Check sheet for the modelled part. Datum: model origin and axes. Units: mm. Give positions to 0.01 mm unless a question says otherwise; leave off trailing zeros. Write each loop counter-clockwise with the first axis right and the second up, starting at its lowest first coordinate (ties: lowest second). Pieces come first, ordered by that corner, then holes. Notation, with made-up numbers: (15.5, 84) -> (49.5, 84) arc R9 cw to (49.5, 91) -> close; hole circle Ø10 at (83.5, -23.75). An arc over 180 degrees is marked (long way). Use a Markdown table: item, result. Add a question column.
1. Cross-section at C-C (z = 10.5). Enter the section's corners in (x, y).
2. Cross-section at A-A (y = -27). Enter the section's corners in (x, z) (3 decimals).
3. Scan lines: probe 1 along Z at (x, y) = (6.35, -19) (3 decimals); probe 2 along X at (y, z) = (-9.5, 0) (3 decimals); probe 3 along Z at (x, y) = (7, -7.5). Record each from-to range of solid material in increasing order. Write a range as [from, to].
4. Cross-section at B-B (z = 34). Enter the section's corners in (x, y).
5. Gauge pin test, flat ends, axial feed: P1, Ø5, axis at y = 3.5, z = 37.5, coming from the +X side; P2, Ø4, axis at x = 6.35, z = -63.5, coming from the -Y side. Record the tip position at first contact, or that the pin passes through.
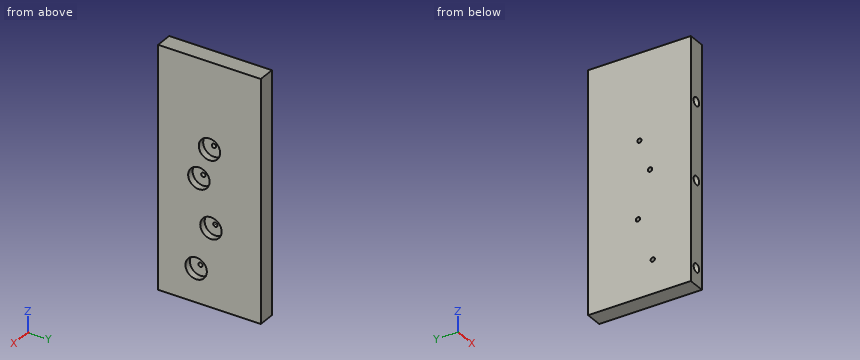
from build123d import *

# Parameters (mm, degrees)
SKETCH1_R                       = 1.5875
SKETCH1_W                       = 25.4
SKETCH1_H                       = 76.2
BOSS_EXTRUDE1_DEPTH             = 12.7
SKETCH2_R                       = 7.9375
CUT_EXTRUDE1_DEPTH              = 5.08
F_1_4_0_25_DIAMETER_HOLE1_D     = 6.35
F_1_4_0_25_DIAMETER_HOLE1_DEPTH = 38.1
F_1_4_0_25_DIAMETER_HOLE1_TIP   = 1.907732465


with BuildPart() as part:
    # Sketch1 → Boss-Extrude1 (new body)
    # profile 1 of 3: a face of its own
    with BuildSketch(Plane(origin=(0, 0, 0), x_dir=(0, 0, -1), z_dir=(1, 0, 0))):
        with BuildLine():
            Line((-76.2, 38.1), (-76.2, 0))
            Line((-76.2, 0), (-39.6875, 0))
            ThreePointArc((-39.6875, 0), (-38.1, 1.5875), (-36.5125, 0))
            Line((-36.5125, 0), (17.574154238, 0))
            ThreePointArc((17.574154238, 0), (18.13214729, 2.569713286), (20.31003158, 1.096077429))
            ThreePointArc((20.31003158, 1.096077429), (20.196167438, 0.505693139), (19.870908922, 0))
            Line((19.870908922, 0), (76.2, 0))
            Line((76.2, 0), (76.2, 38.1))
            Line((76.2, 38.1), (-76.2, 38.1))
        make_face()
    # profile 2 of 3: a face of its own
    with BuildSketch(Plane(origin=(0, 0, 0), x_dir=(0, 0, -1), z_dir=(1, 0, 0))):
        with BuildLine():
            Line((-39.6875, 0), (-76.2, 0))
            Line((-76.2, 0), (-76.2, -38.1))
            Line((-76.2, -38.1), (76.2, -38.1))
            Line((76.2, -38.1), (76.2, 0))
            Line((76.2, 0), (19.870908922, 0))
            ThreePointArc((19.870908922, 0), (18.72253158, -0.491422571), (17.574154238, 0))
            Line((17.574154238, 0), (-36.5125, 0))
            ThreePointArc((-36.5125, 0), (-38.1, -1.5875), (-39.6875, 0))
        make_face()
        with Locations((-14.571224015, -7.860160654)):
            Circle(SKETCH1_R, mode=Mode.SUBTRACT)
        with Locations((51.408255992, -9.873506971)):
            Circle(SKETCH1_R, mode=Mode.SUBTRACT)
    # profile 3 of 3: a face of its own
    with BuildSketch(Plane(origin=(0, 0, 0), x_dir=(0, 0, -1), z_dir=(1, 0, 0))):
        with Locations((-88.9, 0)):
            Rectangle(SKETCH1_W, SKETCH1_H)
    extrude(amount=BOSS_EXTRUDE1_DEPTH)

    # Sketch2 → Cut-Extrude1 (cut)
    with BuildSketch(Plane.ZY.offset(-12.7)):
        with Locations((38.1, 0)):
            Circle(SKETCH2_R)
        with Locations((14.571224015, -7.860160654)):
            Circle(SKETCH2_R)
        with Locations((-18.72253158, 1.096077429)):
            Circle(SKETCH2_R)
        with Locations((-51.408255992, -9.873506971)):
            Circle(SKETCH2_R)
    extrude(amount=CUT_EXTRUDE1_DEPTH, mode=Mode.SUBTRACT)

    # 1_4 _0.25_ Diameter Hole1
    with Locations(Plane.XZ.offset(38.1)):
        with Locations((6.35, -63.5), (6.35, 0), (6.35, 57.15)):
            Hole(F_1_4_0_25_DIAMETER_HOLE1_D / 2, depth=F_1_4_0_25_DIAMETER_HOLE1_DEPTH)
            with Locations((0, 0, -(F_1_4_0_25_DIAMETER_HOLE1_DEPTH + F_1_4_0_25_DIAMETER_HOLE1_TIP / 2))):  # 118° drill point
                Cone(0, F_1_4_0_25_DIAMETER_HOLE1_D / 2, F_1_4_0_25_DIAMETER_HOLE1_TIP, mode=Mode.SUBTRACT)


solid = part.part
Worked answers:
| question | item | result |
|---|---|---|
| 1 | outline | (0, -38.1) -> (12.7, -38.1) -> (12.7, -14.67) -> (7.62, -14.67) -> (7.62, -1.05) -> (12.7, -1.05) -> (12.7, 38.1) -> (0, 38.1) -> close |
| 2 | outline | (0, -76.2) -> (12.7, -76.2) -> (12.7, 101.6) -> (0, 101.6) -> close; hole circle Ø6.35 at (6.35, -63.5); hole circle Ø6.35 at (6.35, 0); hole circle Ø6.35 at (6.35, 57.15) |
| 3 | probe 1 | z = [-76.2, -66.675], [-60.325, -3.175], [3.175, 53.975], [60.325, 101.6] |
| 3 | probe 2 | x = [0, 3.175], [9.525, 12.7] |
| 3 | probe 3 | z = [-76.2, -66.61], [-60.39, -3.11], [3.11, 13.03], [16.12, 54.04], [60.26, 101.6] |
| 4 | outline | (0, -38.1) -> (12.7, -38.1) -> (12.7, -6.8) -> (7.62, -6.8) -> (7.62, 6.8) -> (12.7, 6.8) -> (12.7, 38.1) -> (0, 38.1) -> close |
| 5 | P1 | stops at x = 7.62 |
| 5 | P2 | stops at y = 0.71 |
